Source: CAD feature listing. Evaluate the final solid. Frame: model axes, mm. Face numbers are marked on the shaded views. A direction names the side the tool comes from. Give positions to 0.01 mm unless a question says otherwise; leave off trailing zeros. Order: outer loops, then holes, each group sorted by start corner. A loop starts at its lowest first (then second) coordinate and runs counter-clockwise, first axis right, second up. Notation, with made-up numbers: (37, 24) -> (70, 24) arc R20 ccw to (70, 52) -> close; hole circle Ø6 at (38, 78.25). An arc over 180 degrees is marked (long way). Use CSV: the item, a comma, the result in double quotes.
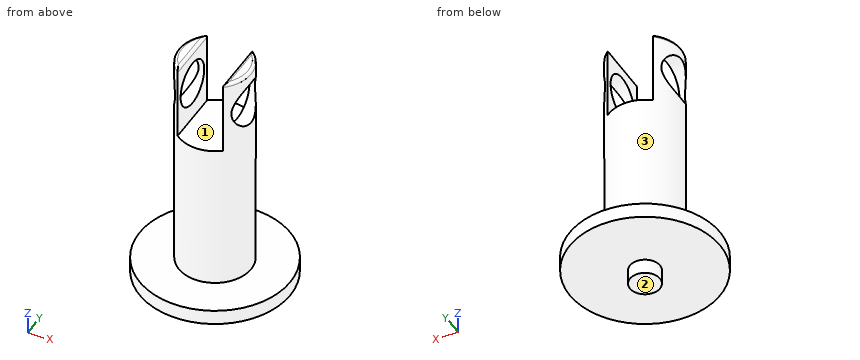
Autodesk Inventor part; units mm, degrees
ref_plane "YZ Plane" through (0, 0, 0) normal (1, 0, 0) x (0, 1, 0)
ref_plane "XZ Plane" through (0, 0, 0) normal (0, 1, 0) x (-1, 0, 0)
ref_plane "XY Plane" through (0, 0, 0) normal (0, 0, 1) x (1, 0, 0)
sketch "Sketch1" plane through (0, 0, 0) normal (0, 0, 1) x (1, 0, 0)
  circle A0 centre (0, 0) radius 250
  dimension "d0" = 500
extrude "Extrusion1" add sketch "Sketch1" along normal blind 50
sketch "Sketch2" plane through (0, 0, 50) normal (0, 0, 1) x (1, 0, 0)
  circle A0 centre (0, 0) radius 120
  dimension "d3" = 240
extrude "Extrusion2" add sketch "Sketch2" along normal blind 750
sketch "Sketch3" plane through (0, 0, 800) normal (0, 0, 1) x (1, 0, 0)
  line L0 (-75, -121) -> (75, -121)
  line L1 (75, -121) -> (75, 121)
  line L2 (75, 121) -> (-75, 121)
  line L3 (-75, 121) -> (-75, -121)
  line L4 (-75, -121) -> (75, 121) construction
  line L5 (75, -121) -> (-75, 121) construction
  point P0 (0, 0)
  dimension "d6" = 150
  dimension "d7" = 150
  dimension "d8" = 121
extrude "Extrusion3" cut sketch "Sketch3" against normal blind 250
sketch "Sketch4" plane through (-75, -93.675, 800) normal (1, 0, 0) x (0, 0, -1)
  circle A0 centre (118.0956, 93.675) radius 75
  point P0 (800, 93.675)
  dimension "d11" = 150
extrude "Extrusion4" cut sketch "Sketch4" along normal mid plane 500
fillet "Fillet1" radius 10 5 edges at (-120, 0, 800) (-75, 0, 800) (75, 0, 800) (108.1665, -51.9615, 800) (108.1665, 51.9615, 800)
sketch "Sketch5" plane through (0, 0, 0) normal (0, 0, -1) x (-1, 0, 0)
  circle A0 centre (0, 0) radius 50
  dimension "d15" = 100
extrude "Extrusion5" add sketch "Sketch5" along normal blind 50
properties part number "Part1final" material "Steel, Carbon"
1. Section query B-B on x = 0. Return loops of the section in (y, z), plus the area to 3 significant figures.
Answer below:
outline,"(-250, 0) -> (-50, 0) -> (-50, -50) -> (50, -50) -> (50, 0) -> (250, 0) -> (250, 50) -> (120, 50) -> (120, 550) -> (-120, 550) -> (-120, 50) -> (-250, 50) -> close"
area,"150,000 mm²"
2. Ray query, line 1 along Z through (x, y) = (89, 0); line 2 along Z through (x, y) = (121.5, 108); line 3 along Y through (x, z) = (84.5, 200.5). Return the intervals inside material, ascending.
Answer below:
line 1,"z = 0 to 606.9, 756.9 to 800"
line 2,"z = 0 to 50"
line 3,"y = -85.2 to 85.2"
3. Section query D-D on z = 449. Return loops of the section in (x, y), plus the area to 3 significant figures.
Answer below:
outline,"circle Ø240 at (0, 0)"
area,"45,200 mm²"
4. Section query C-C on y = 105.5. Return loops of the section in (x, z), plus the area to 3 significant figures.
Answer below:
outline,"(-226.65, 0) -> (226.65, 0) -> (226.65, 50) -> (57.18, 50) -> (57.18, 550) -> (-57.18, 550) -> (-57.18, 50) -> (-226.65, 50) -> close"
area,"79,800 mm²"
5. Access query for the marked faces 1, 2 and 3. Directions: +Z, -Z, +X, -X, +Y, -Y. A direction counts if a zero-diameter tool reaches every point of the face in a straight line with its end or side. Return the directions, or none.
Answer below:
face 1,"+Z, +Y, -Y"
face 2,"-Z, +X, -X, +Y, -Y"
face 3,"+Z"
6. Section query A-A on y = 0. Return loops of the section in (x, z).
Answer below:
outline,"(-250, 0) -> (-50, 0) -> (-50, -50) -> (50, -50) -> (50, 0) -> (250, 0) -> (250, 50) -> (120, 50) -> (120, 606.9) -> (75, 606.9) -> (75, 550) -> (-75, 550) -> (-75, 606.9) -> (-120, 606.9) -> (-120, 50) -> (-250, 50) -> close; (-120, 756.9) -> (-75, 756.9) -> (-75, 790) arc R10 ccw to (-85, 800) -> (-110, 800) arc R10 ccw to (-120, 790) -> close; (75, 756.9) -> (120, 756.9) -> (120, 790) arc R10 ccw to (110, 800) -> (85, 800) arc R10 ccw to (75, 790) -> close"
7. Pin query (flat end, axial travel): P1, Ø4, axis at x = -62.5, y = -91, coming from the +Z side; P2, Ø12, axis at y = -51.5, z = 515.5, coming from the -X side; P3, Ø2, axis at x = 11, y = 77.5, coming from the -Z side. Return the tip coordinate at first contact, or that it passes through.
Answer below:
P1,"stops at z = 550"
P2,"stops at x = -111.04"
P3,"stops at z = 0"
